Build history of the part. All positions in model axes, mm. A direction names the side the tool comes from. Give positions to 0.01 mm unless a question says otherwise; leave off trailing zeros. Write each loop counter-clockwise with the first axis right and the second up, starting at its lowest first coordinate (ties: lowest second). Pieces come first, ordered by that corner, then holes. Notation, with made-up numbers: (62.5, 33) -> (85.5, 33) arc R21 ccw to (85.5, 40) -> close; hole circle Ø6 at (59.25, 43.5). An arc over 180 degrees is marked (long way). One line per question, with ' | ' between items. Start each with the question number.
(1) Tool access for faces 5 (the flat face through (-26, -11.108, 7)), 6 (the flat face through (-76.325, -40, 7)), 7 (the flat face through (-9.025, -15, 7)), 8 (the flat face through (23.675, -40, 7)), 9 (the cylindrical face through (-69.28, -61.26, 13.03)): list every direction of +Z, -Z, +X, -X, +Y, -Y with a clear straight run to the whole face (end or side of a thin tool).
(2) Band-saw the part on C-C, the plane y = -22. Give the cut face in (x, z).
(3) Pin check, flat tips, straight feed: P1, Ø3.5, axis at x = -74.5, y = -62, coming from the +Z side; P2, Ø3.5, axis at x = -40.5, z = 8, coming from the +Y side; P3, Ø5.5, axis at x = -72.83, y = -61.11, coming from the +Z side; P4, Ø6.5, axis at x = 28, z = 6.5, coming from the -Y side. Stop position of each tip, or through.
(4) Drill centre lines: probe 1 along X at (y, z) = (-18, 8.5); probe 2 along Y at (x, z) = (-58, 13.5); probe 3 along X at (y, z) = (-59.5, 4.75). Where is each one in solid material? Low to high. Write a range as from..to.
(5) Band-saw the part on D-D, the plane y = -42. Give the cut face in (x, z), and give its area (3 significant figures).
(6) Pull direction Y, two halves, no side cores. Call faces 1 (the flat face through (-43.625, -15, 7)), 2 (the cylindrical face through (-70.87, -60.49, 5.42)), 3 (the flat face through (-27, -66.108, 7)), 4 (the cylindrical face through (-27, -51, 12)): released by +Y, released by -Y, zero draft, split by the parting line, or undercut.
(7) Band-saw the part on B-B, the plane x = -29.5. Give the cut face in (y, z).
(8) Band-saw the part on A-A, the plane z = 13.5. Count the separate pieces of the cut face and the enclosed holes in it, and give its area (3 significant figures).
from build123d import *

# Parameters (mm, degrees)
F0_R     = 2.05
F1_DEPTH = 15
F2_R     = 3
F3_DEPTH = 121
F4_R     = 3.55
F4_R_2   = 2.05
F5_DEPTH = 4


with BuildPart() as f1:
    # F0 (on Top) → F1 (new body)
    with BuildSketch(Plane.XY):
        Polygon((-43.625293, -11.107708), (-82.325293, -11.107708), (-82.325293, -14.107708), (-76.325293, -14.107708), (-76.325293, -66.107708), (23.674707, -66.107708), (23.674707, -14.107708), (29.674707, -14.107708), (29.674707, -11.107708), (-9.025293, -11.107708), (-9.025293, -19.607708), (-21.325293, -19.607708), (-21.325293, -11.107708), (-31.325293, -11.107708), (-31.325293, -19.607708), (-43.625293, -19.607708), align=None)
        with Locations((-72.825293, -61.107708)):
            Circle(F0_R, mode=Mode.SUBTRACT)
        with Locations((20.174707, -61.107708)):
            Circle(F0_R, mode=Mode.SUBTRACT)
    extrude(amount=F1_DEPTH)

    # F2 (on face) → F3 (cut)
    with BuildSketch(Plane(origin=(-76.325293, 0, 0), x_dir=(0, -1, 0), z_dir=(-1, 0, 0))):
        with Locations((29.107708, 15)):
            Circle(F2_R)
        with Locations((51.107708, 15)):
            Circle(F2_R)
        with Locations((40.107708, 15)):
            Circle(F2_R)
    extrude(amount=-F3_DEPTH, mode=Mode.SUBTRACT)

    # F4 (on face) → F5 (cut)
    with BuildSketch(Plane.XY.offset(15)):
        with Locations((-72.825293, -61.107708)):
            Circle(F4_R)
        with Locations((-72.825293, -61.107708)):
            Circle(F4_R_2, mode=Mode.SUBTRACT)
    extrude(amount=-F5_DEPTH, mode=Mode.SUBTRACT)


solid = f1.part
Results:
1) face 5: +Z, -Z, +X, -X, +Y | face 6: +Z, -Z, -X, -Y | face 7: +Z, -Z, +Y | face 8: +Z, -Z, +X, -Y | face 9: +Z
2) outline: (-76.33, 0) -> (23.67, 0) -> (23.67, 15) -> (-76.33, 15) -> close
3) P1: stops at z = 15 | P2: stops at y = -19.61 | P3: stops at z = 11 | P4: stops at y = -14.11
4) probe 1: x = -76.33..-43.63, -31.33..-21.33, -9.03..23.67 | probe 2: y = -66.11..-53.71, -48.51..-42.71, -37.51..-31.71, -26.51..-11.11 | probe 3: x = -76.33..-74.1, -71.55..18.9, 21.45..23.67
5) outline: (-76.33, 0) -> (23.67, 0) -> (23.67, 12.67) -> (-76.33, 12.67) -> close | area: 1,270 mm²
6) face 1: zero draft | face 2: undercut | face 3: released by -Y | face 4: undercut
7) outline: (-66.11, 0) -> (-11.11, 0) -> (-11.11, 15) -> (-26.11, 15) arc R3 cw to (-32.11, 15) -> (-37.11, 15) arc R3 cw to (-43.11, 15) -> (-48.11, 15) arc R3 cw to (-54.11, 15) -> (-66.11, 15) -> close
8) separate pieces: 4 | enclosed holes: 1 | area: 3,720 mm²
